```python
from build123d import *

# Parameters (mm, degrees)
F1_DEPTH = 25.4
F3_DEPTH = 25.4
F4_W     = 25.4
F4_H     = 25.4
F4_R     = 12.132292
F4_R_2   = 5.440565
F5_DEPTH = 25.4
F7_DEPTH = 25.4
F9_DEPTH = 25.4


with BuildPart() as f1:
    # F0 (on Front) → F1 (new body)
    with BuildSketch(Plane.XZ):
        Polygon((-6.258154, 24.359922), (-31.658154, 24.359922), (-31.658154, -13.740078), (44.541846, -13.740078), (44.541846, -1.040078), (-6.258154, -1.040078), align=None)
    extrude(amount=F1_DEPTH)

    # F2 (on face) → F3 (cut)
    with BuildSketch(Plane.XY.offset(-1.040078)):
        with BuildLine():
            ThreePointArc((32.971398, 0), (44.350376, -13.228424), (31.847373, -25.4))
            Line((31.847373, -25.4), (44.541846, -25.4))
            Line((44.541846, -25.4), (44.541846, 0))
            Line((44.541846, 0), (32.971398, 0))
        make_face()
    extrude(amount=-F3_DEPTH, mode=Mode.SUBTRACT)

    # F4 (on face) → F5 (cut)
    with BuildSketch(Plane.XY.offset(24.359922)):
        with Locations((-18.958154, -12.7)):
            Rectangle(F4_W, F4_H)
        with Locations((-18.958154, -12.7)):
            Circle(F4_R, mode=Mode.SUBTRACT)
        with Locations((-18.958154, -12.7)):
            Circle(F4_R_2)
    extrude(amount=-F5_DEPTH, mode=Mode.SUBTRACT)

    # F6 (on face) → F7 (cut)
    with BuildSketch(Plane.XY.offset(-1.040078)):
        with BuildLine():
            Line((-23.493964, 0), (-31.658154, 0))
            Line((-31.658154, 0), (-31.658154, -25.4))
            Line((-31.658154, -25.4), (-21.405611, -25.4))
            ThreePointArc((-21.405611, -25.4), (-31.43432, -13.438696), (-23.493964, 0))
        make_face()
    extrude(amount=-F7_DEPTH, mode=Mode.SUBTRACT)

    # F8 (on face) → F9 (cut)
    with BuildSketch(Plane.XY.offset(-1.040078)):
        with BuildLine():
            Line((28.453799, -7.700799), (2.349396, -7.700799))
            ThreePointArc((2.349396, -7.700799), (-2.926734, -11.282122), (1.827309, -15.532121))
            Line((1.827309, -15.532121), (28.453799, -15.532121))
            ThreePointArc((28.453799, -15.532121), (32.36946, -11.61646), (28.453799, -7.700799))
        make_face()
    extrude(amount=-F9_DEPTH, mode=Mode.SUBTRACT)


solid = f1.part
```
Check sheet for the modelled part. Datum: model origin and axes. Units: mm. A direction names the side the tool comes from. Round coordinates to 2 decimals unless told otherwise and drop trailing zeros. Loops run counter-clockwise (first coordinate to the right, second up) from the corner with the lowest first, then second, coordinate; pieces in that order, holes last. Notation, with made-up numbers: (66.5, 12.5) - (115.5, 12.5) arc R11 ccw to (115.5, 29.5) - close; hole circle Ø11 at (33, 76). An arc over 180 degrees is marked (long way). Write item = value, one per line. Start each with the question number.
Q1. Depth check by flat-ended pin: P1, Ø1.5, axis at x = -10, z = 3, coming from the -Y side; P2, Ø1, axis at y = -16, z = 16, coming from the +X side; P3, Ø7.5, axis at x = -1.5, y = -8.5, coming from the +Z side. Enter the tip coordinate at first touch or a pass-through.
Q2. Section check D-D (x = -14.5). Record the boundary of the cut face in (y, z), plus the area to 3 significant figures.
Q3. Thickness scan on L1, parallel to Y at x = 25.5, z = -11; L2, parallel to Z at x = 41.5, y = -9.5; L3, parallel to X at y = -11, z = -8. Record the ranges inside material, lowest first.
Q4. Release check for a two-part mould opening along Y. For faces 4 (the face through (-24.2, -15.2, 24.36)), 5 (the face through (15, -15.532, -7)), 6 (the face through (-2.92, -11.18, -7.3)), 7 (the face through (-21.588, -24.544, 11.838)) record: pulls with the +Y half, pulls with the -Y half, needs draft (parallel to the pull), parting line crosses it, or undercut.
Q5. Access from +Z, -Z, +X, -X, +Y, -Y to the whole of each face (thin tool, end or side, straight path). Record for faces 1 (the face through (-19, -13, -1.04)), 2 (the face through (4, 0, -7)), 3 (the face through (16, -7.701, -7)).
Q6. Section check A-A (x = 25.5). Record the boundary of the cut face in (y, z), plus the area to 3 significant figures.
Q7. Section check B-B (z = -9). Record the boundary of the cut face in (x, y).
Q8. Section check C-C (y = -8.75). Record the boundary of the cut face in (x, z), plus the area to 3 significant figures.
Derived:
q1.P1 = -21.63
q1.P2 = -7.15
q1.P3 = -1.04
q2.outline = (-25.4, -13.74) - (0, -13.74) - (0, -1.04) - (-1.42, -1.04) - (-1.42, 24.36) - (-9.58, 24.36) - (-9.58, -1.04) - (-15.82, -1.04) - (-15.82, 24.36) - (-23.98, 24.36) - (-23.98, -1.04) - (-25.4, -1.04) - close
q2.area = 737 mm^2
q3.L1 = -25.4 to -15.53, -7.7 to 0
q3.L2 = -13.74 to -1.04
q3.L3 = -31.41 to -2.9, 32.32 to 44.25
q4.face_4 = needs draft
q4.face_5 = undercut
q4.face_6 = undercut
q4.face_7 = parting line crosses it
q5.face_1 = +Z
q5.face_2 = +Z, -Z, +X, -X, +Y
q5.face_3 = +Z, -Z
q6.outline = (-25.4, -13.74) - (-15.53, -13.74) - (-15.53, -1.04) - (-25.4, -1.04) - close; (-7.7, -13.74) - (0, -13.74) - (0, -1.04) - (-7.7, -1.04) - close
q6.area = 223 mm^2
q7.outline = (-23.49, 0) arc R13.51 ccw to (-21.41, -25.4) - (31.85, -25.4) arc R12.74 ccw to (32.97, 0) - close; hole (1.83, -15.53) - (28.45, -15.53) arc R3.92 ccw to (28.45, -7.7) - (2.35, -7.7) arc R4.05 ccw (long way) to start
q8.outline = (-31, -13.74) - (-1.81, -13.74) - (-1.81, -1.04) - (-7.49, -1.04) - (-7.49, 24.36) - (-15.22, 24.36) - (-15.22, -1.04) - (-22.7, -1.04) - (-22.7, 24.36) - (-30.43, 24.36) - (-30.43, -1.04) - (-31, -1.04) - close; (31.12, -13.74) - (43.75, -13.74) - (43.75, -1.04) - (31.12, -1.04) - close
q8.area = 924 mm^2
